Check sheet for the drawn part. Datum: minimum x, y, z corner. Units: mm. Round coordinates to 2 decimals unless told otherwise and drop trailing zeros. Write each loop counter-clockwise with the first axis right and the second up, starting at its lowest first coordinate (ties: lowest second). Pieces come first, ordered by that corner, then holes. Notation, with made-up numbers: M -32.75,6.25 L 22.25,6.25 A28 ccw 22.25,28.25 Z; hole C -13,71.5 d10. An arc over 180 degrees is marked long. Use a Markdown table: item, result.
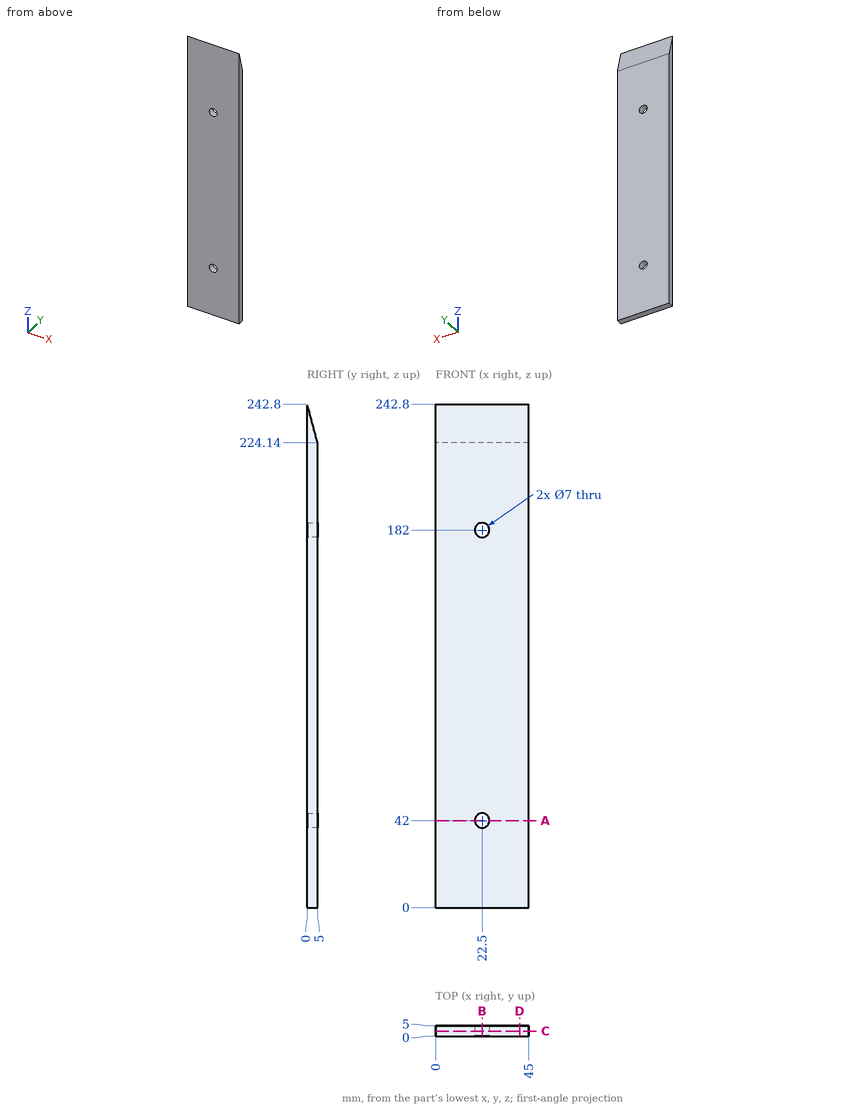
Item 1: Go/stop test with a flat-tipped pin: pin 1 (6.5 mm diameter, centred on x = 22.5, z = 42, fed in from -Y). Record where the tip stops, or that it passes through.
Outcome:
| item | result |
|---|---|
| pin 1 | passes through |
Item 2: Material ranges on line 1 along X through (y, z) = (4, 182); line 2 along Y through (x, z) = (12.5, 227), recorded low to high. Write a range as from..to.
Outcome:
| item | result |
|---|---|
| line 1 | x = 0..19, 26..45 |
| line 2 | y = 0..4.23 |
Item 3: Cross-section at D-D, the plane x = 40.5. Record the cut outline in (y, z), and give its area (3 significant figures).
Outcome:
| item | result |
|---|---|
| outline | M 0,0 L 5,0 L 5,224.14 L 0,242.8 Z |
| area | 1,170 mm2 |
Item 4: Cross-section at C-C, the plane y = 2.35. Record the cut outline in (x, z).
Outcome:
| item | result |
|---|---|
| outline | M 0,0 L 45,0 L 45,234.03 L 0,234.03 Z; hole C 22.5,42 d7; hole C 22.5,182 d7 |
Item 5: Cross-section at B-B, the plane x = 22.5. Record the cut outline in (y, z), and give its area (3 significant figures).
Outcome:
| item | result |
|---|---|
| outline | M 0,0 L 5,0 L 5,38.5 L 0,38.5 Z; M 0,45.5 L 5,45.5 L 5,178.5 L 0,178.5 Z; M 0,185.5 L 5,185.5 L 5,224.14 L 0,242.8 Z |
| area | 1,100 mm2 |
Item 6: Cross-section at A-A, the plane z = 42. Record the cut outline in (x, y).
Outcome:
| item | result |
|---|---|
| outline | M 0,0 L 19,0 L 19,5 L 0,5 Z; M 26,0 L 45,0 L 45,5 L 26,5 Z |
